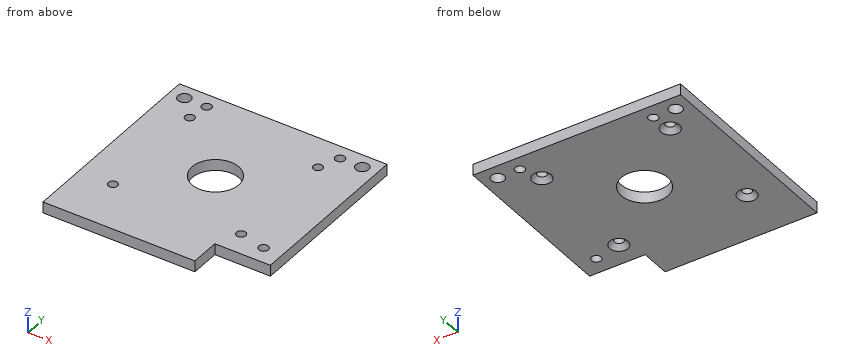
from build123d import *

# Parameters (mm, degrees)
CROQUIS1_W              = 56
CROQUIS1_H              = 55
SALIENTE_EXTRUIR1_DEPTH = 3
CROQUIS2_R              = 1.3
CROQUIS2_W              = 15
CROQUIS2_H              = 8
CROQUIS2_R_2            = 1.75
CORTAR_EXTRUIR1_DEPTH   = 4
CORTAR_EXTRUIR2_REACH   = 42.441
CROQUIS3_R              = 6.3
CROQUIS4_R              = 1.25
CORTAR_EXTRUIR3_DEPTH   = 10
CHAFL_N2_SIZE           = 1.25


with BuildPart() as part:
    # Croquis1 → Saliente-Extruir1 (new body)
    with BuildSketch(Plane.XY):
        with Locations((1.5, 0)):
            Rectangle(CROQUIS1_W, CROQUIS1_H)
    extrude(amount=SALIENTE_EXTRUIR1_DEPTH)

    # Croquis2 → Cortar-Extruir1 (cut)
    with BuildSketch(Plane.XY.offset(3)):
        with Locations((24.5, -14.75)):
            Circle(CROQUIS2_R)
        with Locations((22, -23.5)):
            Rectangle(CROQUIS2_W, CROQUIS2_H)
        with Locations((25.5, 23.528824725)):
            Circle(CROQUIS2_R_2)
        with Locations((19.5, 23.528824725)):
            Circle(CROQUIS2_R)
        with Locations((-22.5, 23.528824725)):
            Circle(CROQUIS2_R_2)
        with Locations((-16.5, 23.528824725)):
            Circle(CROQUIS2_R)
    extrude(amount=-CORTAR_EXTRUIR1_DEPTH, mode=Mode.SUBTRACT)

    # Croquis3 → Cortar-Extruir2 (cut, up to next)
    with BuildSketch(Plane(origin=(0, 0, 0), x_dir=(-1, 0, 0), z_dir=(0, 0, -1)), mode=Mode.PRIVATE) as cortar_extruir2_sk1:
        with Locations((0, 2.414991539)):
            Circle(CROQUIS3_R)
    cortar_extruir2_tool1 = extrude(cortar_extruir2_sk1.sketch, amount=-CORTAR_EXTRUIR2_REACH, mode=Mode.PRIVATE) & part.part
    add(cortar_extruir2_tool1.solids().sort_by_distance((0, 2.414992, 0))[0], mode=Mode.SUBTRACT)

    # Croquis4 → Cortar-Extruir3 (cut)
    with BuildSketch(Plane.XY.offset(3)):
        with Locations((-17.3, 17.914991539)):
            Circle(CROQUIS4_R)
        with Locations((17.3, 17.914991539)):
            Circle(CROQUIS4_R)
        with Locations((-17.3, -13.085008461)):
            Circle(CROQUIS4_R)
        with Locations((17.3, -13.085008461)):
            Circle(CROQUIS4_R)
    extrude(amount=-CORTAR_EXTRUIR3_DEPTH, mode=Mode.SUBTRACT)

    # Chaflán2
    chafl_n2_edges = [part.edges().sort_by_distance(p)[0] for p in [
        (16.05, 17.914991539, 0),
        (-18.55, -13.085008461, 0),
        (16.05, -13.085008461, 0),
        (-18.55, 17.914991539, 0),
    ]]
    chamfer(chafl_n2_edges, length=CHAFL_N2_SIZE)


solid = part.part
Verification items for the finished model (mm, model axes). Coordinates: 2 decimals unless noted, no trailing zeros. Write each loop counter-clockwise with the first axis right and the second up, starting at its lowest first coordinate (ties: lowest second). Pieces come first, ordered by that corner, then holes. Notation, with made-up numbers: (-9, 35.5) - (8, 35.5) arc R19 cw to (8, 55.5) - close; hole circle Ø3 at (-12.75, 20). An arc over 180 degrees is marked (long way). Answer as a JSON object with one key per item and string values.
(1) Cross-section at B-B on x = 17.3. Record the cut outline in (y, z) (3 decimals).
Report:
{"outline": "(-19.5, 0) - (-15.585, 0) - (-14.335, 1.25) - (-14.335, 3) - (-19.5, 3) - close; (-11.835, 1.25) - (-10.585, 0) - (15.415, 0) - (16.665, 1.25) - (16.665, 3) - (-11.835, 3) - close; (19.165, 1.25) - (20.415, 0) - (27.5, 0) - (27.5, 3) - (19.165, 3) - close"}
(2) Cross-section at A-A on x = 0. Record the cut outline in (y, z) (3 decimals), plus the area to 3 significant figures.
Report:
{"outline": "(-27.5, 0) - (-3.885, 0) - (-3.885, 3) - (-27.5, 3) - close; (8.715, 0) - (27.5, 0) - (27.5, 3) - (8.715, 3) - close", "area": "127 mm^2"}
(3) Cross-section at D-D on y = 7.5. Record the cut outline in (x, z).
Report:
{"outline": "(-26.5, 0) - (-3.72, 0) - (-3.72, 3) - (-26.5, 3) - close; (3.72, 0) - (29.5, 0) - (29.5, 3) - (3.72, 3) - close"}
(4) Gauge pin test, flat ends, axial feed: pin 1 Ø2 at (x, y) = (17.3, -13.09) entering from -Z; pin 2 Ø1.5 at (x, z) = (22, 1) entering from -Y. Record the tip position at first contact, or that the pin passes through.
Report:
{"pin 1": "through", "pin 2": "y = -19.5"}
(5) Thickness scan on line 1 along Y through (x, z) = (17.5, 2.65); line 2 along Y through (x, z) = (-22.5, 0.7); line 3 along Y through (x, z) = (17.3, 2.55) (3 decimals). Record the ranges inside material, lowest first.
Report:
{"line 1": "-19.5 to -14.32, -11.85 to 16.68, 19.15 to 27.5", "line 2": "-27.5 to 21.78, 25.28 to 27.5", "line 3": "-19.5 to -14.335, -11.835 to 16.665, 19.165 to 27.5"}
(6) Cross-section at C-C on z = 2.05. Give the number of separate pieces and of enclosed holes in the cut face, plus the area to 3 significant figures.
Report:
{"separate pieces": "1", "enclosed holes": "10", "area": "2,780 mm^2"}
